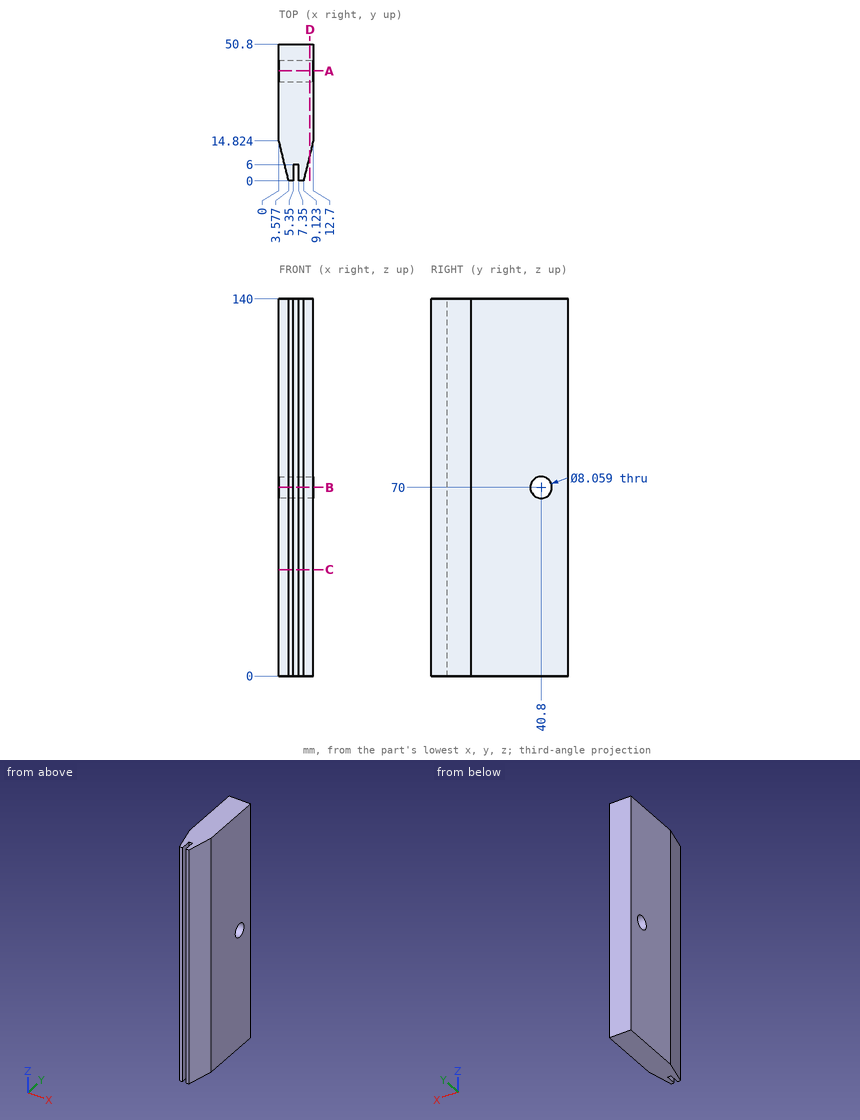
Part print with two shaded views. Sizes in mm from the minimum x, y, z corner. Coordinates: 2 decimals unless noted, no trailing zeros. Order: outer loops, then holes, each group sorted by start corner. A loop starts at its lowest first (then second) coordinate and runs counter-clockwise, first axis right, second up. Notation, with made-up numbers: M 12.25,-25 L 63.25,-25 A9 cw 63.25,-9 Z; hole C -27,56 d5. An arc over 180 degrees is marked long. One line per question, with ' | ' between items. Start each with the question number.
1. Cut at D-D (x = 11.5). Write the cut outline in (y, z), plus the area to 3 significant figures.
2. Cut at A-A (y = 40.8). Write the cut outline in (x, z).
3. Cut at B-B (z = 70). Write the cut outline in (x, y).
4. Flat gauge pins, fed straight in: P1, Ø0.6, axis at x = 6, z = 82.5, coming from the -Y side; P2, Ø5, axis at y = 4, z = 92, coming from the +X side; P3, Ø6.5, axis at y = 4, z = 85, coming from the -X side. Where does each tip first touch, or does it go through?
5. Cut at C-C (z = 39.5). Write the cut outline in (x, y), plus the area to 3 significant figures.
6. Wall check: line 1 along Z through (x, y) = (4.5, 41) (1 decimal); line 2 along Y through (x, z) = (8, 70); line 3 along Y through (x, z) = (6, 70). Give the ranges that are in metal, low to high. Write a range as [from, to].
The answers:
1) outline: M 9.85,0 L 50.8,0 L 50.8,140 L 9.85,140 Z; hole C 40.8,70 d8.06 | area: 5,680 mm2
2) outline: M 0,0 L 12.7,0 L 12.7,65.97 L 0,65.97 Z; M 0,74.03 L 12.7,74.03 L 12.7,140 L 0,140 Z
3) outline: M 0,14.82 L 3.58,0 L 5.35,0 L 5.35,6 L 7.35,6 L 7.35,0 L 9.12,0 L 12.7,14.82 L 12.7,36.77 L 0,36.77 Z; M 0,44.83 L 12.7,44.83 L 12.7,50.8 L 0,50.8 Z
4) P1: stops at y = 6 | P2: stops at x = 10.69 | P3: stops at x = 1.83
5) outline: M 0,14.82 L 3.58,0 L 5.35,0 L 5.35,6 L 7.35,6 L 7.35,0 L 9.12,0 L 12.7,14.82 L 12.7,50.8 L 0,50.8 Z | area: 580 mm2
6) line 1: z = [0, 66], [74, 140] | line 2: y = [0, 36.77], [44.83, 50.8] | line 3: y = [6, 36.77], [44.83, 50.8]
